from build123d import *

# Parameters (mm, degrees)
F0_R     = 63.0332735131
F0_R_2   = 50.1119097805
F1_DEPTH = 25.4
F2_DEPTH = 25.4
F3_W     = 148.2297182083
F3_H     = 88.6540859938
F4_DEPTH = 25.4
F5_DEPTH = 25.4


with BuildPart() as f1:
    # F0 (on Front) → F1 (new body)
    with BuildSketch(Plane.XZ):
        with Locations((-0.360891223, 0.7217377424)):
            Circle(F0_R)
        Circle(F0_R_2, mode=Mode.SUBTRACT)
    extrude(amount=F1_DEPTH)

    # F2 (add): a face of the model
    f2_faces = [f1.faces().sort_by_distance(p)[0] for p in [
        (-61.6113145304, -25.4, 0.7217377424),
    ]]
    extrude(f2_faces, amount=F2_DEPTH)

    # F3 (on Front) → F4 (join)
    with BuildSketch(Plane.XZ):
        with Locations((-62.5252425671, 0)):
            Rectangle(F3_W, F3_H)
    extrude(amount=F4_DEPTH)

    # F5 (cut): a face of the model
    f5_faces = [f1.faces().sort_by_distance(p)[0] for p in [
        (-15.9361897378, -25.4, 0),
    ]]
    extrude(f5_faces, amount=-F5_DEPTH, mode=Mode.SUBTRACT)


solid = f1.part
Model file for the job. Use its own axes, mm. A direction names the side the tool comes from. Give positions to 0.01 mm unless a question says otherwise; leave off trailing zeros. Loops run counter-clockwise (first coordinate to the right, second up) from the corner with the lowest first, then second, coordinate; pieces in that order, holes last.
1) Flat gauge pins, fed straight in: pin 1 Ø7.5 at (x, y) = (-73.5, -12) entering from +Z; pin 2 Ø2 at (x, z) = (-72.5, -15.5) entering from -Y; pin 3 Ø6 at (y, z) = (-45, 27.5) entering from +X. Where does each tip first touch, or does it go through?
2) Saw through at B-B (z = -33). Write the cut outline in (x, y).
3) Wall check: line 1 (Z direction, x = 0, y = -15); line 2 (X direction, y = -39, z = -9). Give the ranges that are in metal, low to high.
4) Saw through at C-C (y = -20). Write the cut outline in (x, z).
5) Tool access for faces 5 (the flat face through (-92, -13, 44.327)), 6 (the flat face through (-43, -50.8, -27)), 7 (the flat face through (-91, -13, -44.327)): list every direction of +Z, -Z, +X, -X, +Y, -Y with a clear straight run to the whole face (end or side of a thin tool).
6) Saw through at A-A (x = -27.5). Write the cut outline in (y, z).
7) Pull direction X, two halves, no side cores. Call faces 1 (the cylindrical face through (-6.524, -25.044, 49.685)), 2 (the flat face through (-136.64, -13, -1)), 3 (the cylindrical face through (59.76, -25.04, 19.66)), 4 (the flat face through (-61, 0, 2)): +X half, -X half, draft (parallel to the pull), parting line (faces both ways), or undercut.
8) Saw through at D-D (x = -6). Write the cut outline in (y, z), plus the area to 3 significant figures.
Answer block:
1. pin 1: stops at z = 44.33
1. pin 2: stops at y = -25.4
1. pin 3: stops at x = 58.02
2. outline: (-136.64, -25.4) - (-53.62, -25.4) - (-53.62, -50.8) - (-37.71, -50.8) - (-37.71, 0) - (-136.64, 0) - close; (37.71, -50.8) - (52.89, -50.8) - (52.89, 0) - (37.71, 0) - close
3. line 1: z = -62.31 to -50.11, 50.11 to 63.75
3. line 2: x = -62.64 to -49.3, 49.3 to 61.92
4. outline: (-136.64, -44.33) - (-44.45, -44.33) arc R63.03 ccw (long way) to (-45.88, 44.33) - (-136.64, 44.33) - close; hole circle Ø100.22 at (0, 0)
5. face 5: +Z, -X, +Y, -Y
5. face 6: +Z, -Z, +X, -X, -Y
5. face 7: -Z, -X, +Y, -Y
6. outline: (-50.8, -56.17) - (0, -56.17) - (0, -41.89) - (-50.8, -41.89) - close; (-50.8, 41.89) - (0, 41.89) - (0, 57.61) - (-50.8, 57.61) - close
7. face 1: undercut
7. face 2: -X half
7. face 3: parting line
7. face 4: draft
8. outline: (-50.8, -62.06) - (0, -62.06) - (0, -49.75) - (-50.8, -49.75) - close; (-50.8, 49.75) - (0, 49.75) - (0, 63.5) - (-50.8, 63.5) - close
8. area: 1,320 mm2
